Read the model definition and answer for the solid it produces. Units are mm, in the model's axes. A direction names the side the tool comes from. Give positions to 0.01 mm unless a question says otherwise; leave off trailing zeros. Order: outer loops, then holes, each group sorted by start corner. A loop starts at its lowest first (then second) coordinate and runs counter-clockwise, first axis right, second up. Notation, with made-up numbers: (-31.5, 46.25) -> (-12.5, 46.25) arc R9 ccw to (-12.5, 57.25) -> close; hole circle Ø6 at (67.5, 53). An arc over 180 degrees is marked (long way). Use one line per item in the form item = value.
```python
from build123d import *

# Parameters (mm, degrees)
BOSS_EXTRUDE3_DEPTH  = 125
SKETCH3_W            = 125
SKETCH3_H            = 69.296464556
BOSS_EXTRUDE5_DEPTH  = 12
CUT_EXTRUDE1_DEPTH   = 159.836393815
SKETCH7_W            = 105
SKETCH7_H            = 10
BOSS_EXTRUDE6_DEPTH  = 8
SKETCH8_W            = 105
SKETCH8_H            = 10
BOSS_EXTRUDE7_DEPTH  = 8
SKETCH9_W            = 105
SKETCH9_H            = 55.154328932
CUT_EXTRUDE2_DEPTH   = 161.78246173
SKETCH11_W           = 10
SKETCH11_H           = 55.154328932
CUT_EXTRUDE3_DEPTH   = 6
SKETCH12_W           = 10
SKETCH12_H           = 55.154328932
CUT_EXTRUDE4_DEPTH   = 6
SKETCH13_W           = 105
SKETCH13_H           = 61.154328932
CUT_EXTRUDE6_DEPTH   = 3
SKETCH14_R           = 1.9
CUT_EXTRUDE8_DEPTH   = 6
SKETCH15_R           = 1.9
CUT_EXTRUDE9_DEPTH   = 6
BOSS_EXTRUDE9_REACH  = 158.4
SKETCH25_W           = 10
SKETCH25_H           = 6
BOSS_EXTRUDE13_DEPTH = 10
CUT_EXTRUDE10_DEPTH  = 1
CUT_EXTRUDE11_DEPTH  = 1
SKETCH29_W           = 11
SKETCH29_H           = 81.296464556
BOSS_EXTRUDE15_DEPTH = 6
SKETCH31_R           = 2
CUT_EXTRUDE16_DEPTH  = 6
SKETCH32_R           = 2
CUT_EXTRUDE17_DEPTH  = 6
CUT_EXTRUDE22_DEPTH  = 157.400127877
CUT_EXTRUDE23_DEPTH  = 157.400127877
CUT_EXTRUDE26_REACH  = 164.072


with BuildPart() as part:
    # Sketch1 → Boss-Extrude3 (new body)
    with BuildSketch(Plane(origin=(0, 0, 0), x_dir=(0, 0, -1), z_dir=(1, 0, 0))):
        Polygon((0, 0), (69.296464556, 0), (0, 69.296464556), align=None)
    extrude(amount=-BOSS_EXTRUDE3_DEPTH)

    # Sketch3 → Boss-Extrude5 (add)
    with BuildSketch(Plane.XZ):
        with Locations((-62.5, -34.648232278)):
            Rectangle(SKETCH3_W, SKETCH3_H)
    extrude(amount=BOSS_EXTRUDE5_DEPTH)

    # Sketch6 → Cut-Extrude1 (cut, through all)
    with BuildSketch(Plane.ZY.offset(125)):
        Polygon((-7.071067812, 62.225396744), (-62.225396744, 7.071067812), (-7.071067812, 7.071067812), align=None)
    extrude(amount=-CUT_EXTRUDE1_DEPTH, mode=Mode.SUBTRACT)

    # Sketch7 → Boss-Extrude6 (add)
    with BuildSketch(Plane(origin=(0, 34.648232278, -34.648232278), x_dir=(1, 0, 0), z_dir=(0, 0.7071067811865515, -0.7071067811865436))):
        with Locations((-62.5, 44)):
            Rectangle(SKETCH7_W, SKETCH7_H)
    extrude(amount=BOSS_EXTRUDE6_DEPTH)

    # Sketch8 → Boss-Extrude7 (add)
    with BuildSketch(Plane(origin=(0, 34.648232278, -34.648232278), x_dir=(1, 0, 0), z_dir=(0, 0.7071067811865515, -0.7071067811865436))):
        with Locations((-62.5, -44)):
            Rectangle(SKETCH8_W, SKETCH8_H)
    extrude(amount=BOSS_EXTRUDE7_DEPTH)

    # Sketch9 → Cut-Extrude2 (cut, through all)
    with BuildSketch(Plane(origin=(0, 7.071067812, 0), x_dir=(1, 0, 0), z_dir=(0, 1, 0))):
        with Locations((-62.5, 34.648232278)):
            Rectangle(SKETCH9_W, SKETCH9_H)
    extrude(amount=-CUT_EXTRUDE2_DEPTH, mode=Mode.SUBTRACT)

    # Sketch11 → Cut-Extrude3 (cut)
    with BuildSketch(Plane(origin=(0, 7.071067812, 0), x_dir=(1, 0, 0), z_dir=(0, 1, 0))):
        with Locations((-5, 34.648232278)):
            Rectangle(SKETCH11_W, SKETCH11_H)
    extrude(amount=-CUT_EXTRUDE3_DEPTH, mode=Mode.SUBTRACT)

    # Sketch12 → Cut-Extrude4 (cut)
    with BuildSketch(Plane(origin=(0, 7.071067812, 0), x_dir=(1, 0, 0), z_dir=(0, 1, 0))):
        with Locations((-120, 34.648232278)):
            Rectangle(SKETCH12_W, SKETCH12_H)
    extrude(amount=-CUT_EXTRUDE4_DEPTH, mode=Mode.SUBTRACT)

    # Sketch13 → Cut-Extrude6 (cut)
    with BuildSketch(Plane(origin=(0, 0, -7.071067812), x_dir=(-1, 0, 0), z_dir=(0, 0, -1))):
        with Locations((62.5, 31.648232278)):
            Rectangle(SKETCH13_W, SKETCH13_H)
    extrude(amount=-CUT_EXTRUDE6_DEPTH, mode=Mode.SUBTRACT)

    # Sketch14 → Cut-Extrude8 (cut)
    with BuildSketch(Plane(origin=(0, 34.648232278, -34.648232278), x_dir=(1, 0, 0), z_dir=(0, 0.7071067811865515, -0.7071067811865436))):
        with Locations(Location((-6.25, 42.75, 0), (0, 0, 270))):
            Circle(SKETCH14_R)
    cut_extrude8 = extrude(amount=-CUT_EXTRUDE8_DEPTH, mode=Mode.SUBTRACT)

    # Mirror1: Cut-Extrude8 across plane
    add(cut_extrude8.mirror(Plane(origin=(-62.5, 0, 0), x_dir=(0, 0, 1), z_dir=(1, 0, 0))), mode=Mode.SUBTRACT)

    # Sketch15 → Cut-Extrude9 (cut)
    with BuildSketch(Plane(origin=(0, 34.648232278, -34.648232278), x_dir=(1, 0, 0), z_dir=(0, 0.7071067811865515, -0.7071067811865436))):
        with Locations(Location((-6.25, -42.75, 0), (0, 0, 270))):
            Circle(SKETCH15_R)
    cut_extrude9 = extrude(amount=-CUT_EXTRUDE9_DEPTH, mode=Mode.SUBTRACT)

    # Mirror2: Cut-Extrude9 across plane
    add(cut_extrude9.mirror(Plane(origin=(-62.5, 0, 0), x_dir=(0, 0, 1), z_dir=(1, 0, 0))), mode=Mode.SUBTRACT)

    # Sketch22 → Boss-Extrude9 (add, up to next)
    with BuildSketch(Plane.ZY.offset(10), mode=Mode.PRIVATE) as boss_extrude9_sk1:
        Polygon((-7.071067812, 62.225396744), (-4.071067812, 59.225396744), (-4.071067812, 62.225396744), align=None)
    boss_extrude9_tool1 = extrude(boss_extrude9_sk1.sketch, amount=BOSS_EXTRUDE9_REACH, mode=Mode.PRIVATE) - part.part
    add(boss_extrude9_tool1.solids().sort_by_distance((-10, 61.225397, -5.071068))[0])

    # Sketch25 → Boss-Extrude13 (add)
    with BuildSketch(Plane.XY.offset(-62.225396744)):
        with Locations((-5, 4.071067812)):
            Rectangle(SKETCH25_W, SKETCH25_H)
        with Locations((-120, 4.071067812)):
            Rectangle(SKETCH25_W, SKETCH25_H)
    extrude(amount=BOSS_EXTRUDE13_DEPTH)

    # Sketch26 → Cut-Extrude10 (cut)
    with BuildSketch(Plane(origin=(-10, 0, 0), x_dir=(0, 0, -1), z_dir=(1, 0, 0))):
        Polygon((0, 69.296464556), (7.071067812, 62.225396744), (12.727922061, 67.882250994), (5.656854249, 74.953318806), align=None)
    cut_extrude10 = extrude(amount=-CUT_EXTRUDE10_DEPTH, mode=Mode.SUBTRACT)

    # Sketch27 → Cut-Extrude11 (cut)
    with BuildSketch(Plane(origin=(-10, 0, 0), x_dir=(0, 0, -1), z_dir=(1, 0, 0))):
        Polygon((62.225396744, 7.071067812), (69.296464556, 0), (74.953318806, 5.656854249), (67.882250994, 12.727922061), align=None)
    cut_extrude11 = extrude(amount=-CUT_EXTRUDE11_DEPTH, mode=Mode.SUBTRACT)

    # Mirror3: Cut-Extrude10, Cut-Extrude11 across plane
    add(cut_extrude10.mirror(Plane(origin=(-62.5, 0, 0), x_dir=(0, 0, 1), z_dir=(1, 0, 0))), mode=Mode.SUBTRACT)
    add(cut_extrude11.mirror(Plane(origin=(-62.5, 0, 0), x_dir=(0, 0, 1), z_dir=(1, 0, 0))), mode=Mode.SUBTRACT)

    # Sketch29 → Boss-Extrude15 (add)
    with BuildSketch(Plane.XY):
        with Locations((-5.5, 28.648232278)):
            Rectangle(SKETCH29_W, SKETCH29_H)
    boss_extrude15 = extrude(amount=BOSS_EXTRUDE15_DEPTH)

    # Mirror4: Boss-Extrude15 across plane
    add(boss_extrude15.mirror(Plane(origin=(-62.5, 0, 0), x_dir=(0, 0, 1), z_dir=(1, 0, 0))))

    # Sketch31 → Cut-Extrude16 (cut)
    with BuildSketch(Plane(origin=(0, 34.648232278, -34.648232278), x_dir=(1, 0, 0), z_dir=(0, 0.7071067811865513, -0.7071067811865438))):
        with Locations(Location((-6.25, 42.75, 0), (0, 0, 270))):
            Circle(SKETCH31_R)
    cut_extrude16 = extrude(amount=-CUT_EXTRUDE16_DEPTH, mode=Mode.SUBTRACT)

    # Sketch32 → Cut-Extrude17 (cut)
    with BuildSketch(Plane(origin=(0, 34.648232278, -34.648232278), x_dir=(1, 0, 0), z_dir=(0, 0.7071067811865513, -0.7071067811865438))):
        with Locations(Location((-6.25, -42.75, 0), (0, 0, 270))):
            Circle(SKETCH32_R)
    cut_extrude17 = extrude(amount=-CUT_EXTRUDE17_DEPTH, mode=Mode.SUBTRACT)

    # Mirror5: Cut-Extrude16, Cut-Extrude17 across plane
    add(cut_extrude16.mirror(Plane(origin=(-62.5, 0, 0), x_dir=(0, 0, 1), z_dir=(1, 0, 0))), mode=Mode.SUBTRACT)
    add(cut_extrude17.mirror(Plane(origin=(-62.5, 0, 0), x_dir=(0, 0, 1), z_dir=(1, 0, 0))), mode=Mode.SUBTRACT)

    # Sketch41 → Cut-Extrude22 (cut, through all)
    with BuildSketch(Plane.ZY.offset(10)):
        Polygon((-7.071067812, 1.071067812), (-4.071067812, 1.071067812), (-4.071067812, 59.225396744), (-7.071067812, 62.225396744), align=None)
    extrude(amount=-CUT_EXTRUDE22_DEPTH, mode=Mode.SUBTRACT)

    # Sketch42 → Cut-Extrude23 (cut, through all)
    with BuildSketch(Plane(origin=(-115, 0, 0), x_dir=(0, 0, -1), z_dir=(1, 0, 0))):
        Polygon((7.071067812, 1.071067812), (4.071067812, 1.071067812), (4.071067812, 59.225396744), (7.071067812, 62.225396744), align=None)
    extrude(amount=-CUT_EXTRUDE23_DEPTH, mode=Mode.SUBTRACT)

    # Sketch43 → Cut-Extrude26 (cut, up to next)
    with BuildSketch(Plane(origin=(0, 0, -4.071067812), x_dir=(-1, 0, 0), z_dir=(0, 0, -1)), mode=Mode.PRIVATE) as cut_extrude26_sk1:
        Polygon((36.748988877, 34.169774937), (58.011664466, 53.225396744), (15.486313289, 53.225396744), align=None)
    cut_extrude26_tool1 = extrude(cut_extrude26_sk1.sketch, amount=-CUT_EXTRUDE26_REACH, mode=Mode.PRIVATE) & part.part
    # Sketch43 → Cut-Extrude26 (cut, up to next)
    with BuildSketch(Plane(origin=(0, 0, -4.071067812), x_dir=(-1, 0, 0), z_dir=(0, 0, -1)), mode=Mode.PRIVATE) as cut_extrude26_sk2:
        Polygon((32.260614543, 30.147291337), (11, 49.201066035), (11, 11.093516639), align=None)
    cut_extrude26_tool2 = extrude(cut_extrude26_sk2.sketch, amount=-CUT_EXTRUDE26_REACH, mode=Mode.PRIVATE) & part.part
    # Sketch43 → Cut-Extrude26 (cut, up to next)
    with BuildSketch(Plane(origin=(0, 0, -4.071067812), x_dir=(-1, 0, 0), z_dir=(0, 0, -1)), mode=Mode.PRIVATE) as cut_extrude26_sk3:
        Polygon((58.009015214, 7.07156019), (36.747854103, 26.125824723), (15.486143585, 7.071067812), (58.008465808, 7.071067812), align=None)
    cut_extrude26_tool3 = extrude(cut_extrude26_sk3.sketch, amount=-CUT_EXTRUDE26_REACH, mode=Mode.PRIVATE) & part.part
    # Sketch43 → Cut-Extrude26 (cut, up to next)
    with BuildSketch(Plane(origin=(0, 0, -4.071067812), x_dir=(-1, 0, 0), z_dir=(0, 0, -1)), mode=Mode.PRIVATE) as cut_extrude26_sk4:
        Polygon((83.760065137, 30.149665598), (62.498904026, 49.20393013), (41.236228437, 30.148308322), (62.497389548, 11.09404379), align=None)
    cut_extrude26_tool4 = extrude(cut_extrude26_sk4.sketch, amount=-CUT_EXTRUDE26_REACH, mode=Mode.PRIVATE) & part.part
    # Sketch43 → Cut-Extrude26 (cut, up to next)
    with BuildSketch(Plane(origin=(0, 0, -4.071067812), x_dir=(-1, 0, 0), z_dir=(0, 0, -1)), mode=Mode.PRIVATE) as cut_extrude26_sk5:
        Polygon((109.511664466, 7.071067812), (88.249757212, 26.126001038), (66.987849957, 7.071067812), align=None)
    cut_extrude26_tool5 = extrude(cut_extrude26_sk5.sketch, amount=-CUT_EXTRUDE26_REACH, mode=Mode.PRIVATE) & part.part
    # Sketch43 → Cut-Extrude26 (cut, up to next)
    with BuildSketch(Plane(origin=(0, 0, -4.071067812), x_dir=(-1, 0, 0), z_dir=(0, 0, -1)), mode=Mode.PRIVATE) as cut_extrude26_sk6:
        Polygon((114, 11.093516639), (114, 49.203383091), (92.738092746, 30.148449865), align=None)
    cut_extrude26_tool6 = extrude(cut_extrude26_sk6.sketch, amount=-CUT_EXTRUDE26_REACH, mode=Mode.PRIVATE) & part.part
    # Sketch43 → Cut-Extrude26 (cut, up to next)
    with BuildSketch(Plane(origin=(0, 0, -4.071067812), x_dir=(-1, 0, 0), z_dir=(0, 0, -1)), mode=Mode.PRIVATE) as cut_extrude26_sk7:
        Polygon((109.508465808, 53.225396744), (66.988335534, 53.225396744), (88.248400671, 34.172114425), align=None)
    cut_extrude26_tool7 = extrude(cut_extrude26_sk7.sketch, amount=-CUT_EXTRUDE26_REACH, mode=Mode.PRIVATE) & part.part
    add(cut_extrude26_tool1.solids().sort_by_distance((-36.748989, 46.873523, -4.071068))[0], mode=Mode.SUBTRACT)
    add(cut_extrude26_tool2.solids().sort_by_distance((-18.086872, 30.147291, -4.071068))[0], mode=Mode.SUBTRACT)
    add(cut_extrude26_tool3.solids().sort_by_distance((-36.747854, 13.422653, -4.071068))[0], mode=Mode.SUBTRACT)
    add(cut_extrude26_tool4.solids().sort_by_distance((-62.498147, 30.148987, -4.071068))[0], mode=Mode.SUBTRACT)
    add(cut_extrude26_tool5.solids().sort_by_distance((-88.249757, 13.422712, -4.071068))[0], mode=Mode.SUBTRACT)
    add(cut_extrude26_tool6.solids().sort_by_distance((-106.912698, 30.14845, -4.071068))[0], mode=Mode.SUBTRACT)
    add(cut_extrude26_tool7.solids().sort_by_distance((-88.248401, 46.874303, -4.071068))[0], mode=Mode.SUBTRACT)


solid = part.part
```
Item 1: Given pin 1 Ø2 at (x, z) = (-30.5, -3.5) entering from +Y; pin 2 Ø1.8 at (x, z) = (-3.5, 3.5) entering from +Y; pin 3 Ø4 at (x, y) = (-76, -2.5) entering from -Z, each flat-ended and moving along its own axis, determine where each tip first touches the part or whether it passes through.
Checks:
pin_1 = 73.8
pin_2 = 69.3
pin_3 = -69.3
Item 2: The part is cut by section A-A on z = -18. Give the vertices of the cut face in (x, y), and give its area (3 significant figures).
Checks:
outline = (-125, -12) -> (-115, -12) -> (-115, 1.07) -> (-125, 1.07) -> close; (-10, -12) -> (0, -12) -> (0, 1.07) -> (-10, 1.07) -> close
area = 261 mm²
Item 3: The part is cut by section D-D on x = -81.5. Give the vertices of the cut face in (y, z), and give its area (3 significant figures).
Checks:
outline = (-12, -69.3) -> (0, -69.3) -> (5.66, -74.95) -> (12.73, -67.88) -> (7.07, -62.23) -> (-12, -62.23) -> close; (-12, -7.07) -> (1.07, -7.07) -> (1.07, -4.07) -> (7.07, -4.07) -> (7.07, 0) -> (-12, 0) -> close; (20.08, -4.07) -> (28.12, -4.07) -> (28.12, 0) -> (20.08, 0) -> close; (32.18, -4.07) -> (40.22, -4.07) -> (40.22, 0) -> (32.18, 0) -> close; (53.23, -4.07) -> (59.23, -4.07) -> (67.88, -12.73) -> (74.95, -5.66) -> (69.3, 0) -> (53.23, 0) -> close
area = 518 mm²
Item 4: The part is cut by section C-C on x = -56. Give the vertices of the cut face in (y, z), and give its area (3 significant figures).
Checks:
outline = (-12, -69.3) -> (0, -69.3) -> (5.66, -74.95) -> (12.73, -67.88) -> (7.07, -62.23) -> (-12, -62.23) -> close; (-12, -7.07) -> (1.07, -7.07) -> (1.07, -4.07) -> (7.07, -4.07) -> (7.07, 0) -> (-12, 0) -> close; (8.87, -4.07) -> (16.92, -4.07) -> (16.92, 0) -> (8.87, 0) -> close; (43.38, -4.07) -> (51.42, -4.07) -> (51.42, 0) -> (43.38, 0) -> close; (53.23, -4.07) -> (59.23, -4.07) -> (67.88, -12.73) -> (74.95, -5.66) -> (69.3, 0) -> (53.23, 0) -> close
area = 518 mm²
Item 5: Straight lines are drawn through the part: L1, parallel to Y at x = -44, z = -1.5; L2, parallel to Y at x = -118, z = -55.5; L3, parallel to Y at x = -55, z = -5. For each, find the intervals that lie inside material, in ascending order. Write a range as from..to.
Checks:
L1 = -12..7.07, 19.63..27.67, 32.63..40.67, 53.23..70.8
L2 = -12..7.07
L3 = -12..1.07, 60.15..74.3
Item 6: Which of the six approach directions +Z, -Z, +X, -X, +Y, -Y give full straight-line access (tool end or side, diameter ignored) to faces 5 (the flat face through (-119.577, 2.799, -66.497)), 6 (the flat face through (-36, 7.071, -2)), 7 (the flat face through (-73.28, 39.54, -2.06)), 8 (the flat face through (-61.625, 63.493, -8.339))?
Checks:
face_5 = -Z, -X, +Y
face_6 = +Z
face_7 = +Z, -Z
face_8 = -Z, +X, -X
Item 7: The part is cut by section B-B on y = 38. Give the vertices of the cut face in (x, z), and give its area (3 significant figures).
Checks:
outline = (-125, -4.07) -> (-114, -4.07) -> (-114, 6) -> (-125, 6) -> close; (-101.5, -4.07) -> (-92.52, -4.07) -> (-92.52, 0) -> (-101.5, 0) -> close; (-83.98, -4.07) -> (-75, -4.07) -> (-75, 0) -> (-83.98, 0) -> close; (-50, -4.07) -> (-41.02, -4.07) -> (-41.02, 0) -> (-50, 0) -> close; (-32.48, -4.07) -> (-23.5, -4.07) -> (-23.5, 0) -> (-32.48, 0) -> close; (-11, -4.07) -> (0, -4.07) -> (0, 6) -> (-11, 6) -> close
area = 368 mm²
Item 8: Determine the mould class of faces 1 (the flat face through (-63, -5, -7.071)), 2 (the flat face through (-63.221, 2.789, -72.085)), 3 (the flat face through (-6, 69.296, 3)), 4 (the flat face through (-6.22, 60.61, -0.2)) for opening direction Y: +Y half, -Y half, draft (parallel to the pull), parting line (faces both ways), or undercut.
Checks:
face_1 = draft
face_2 = -Y half
face_3 = +Y half
face_4 = undercut
